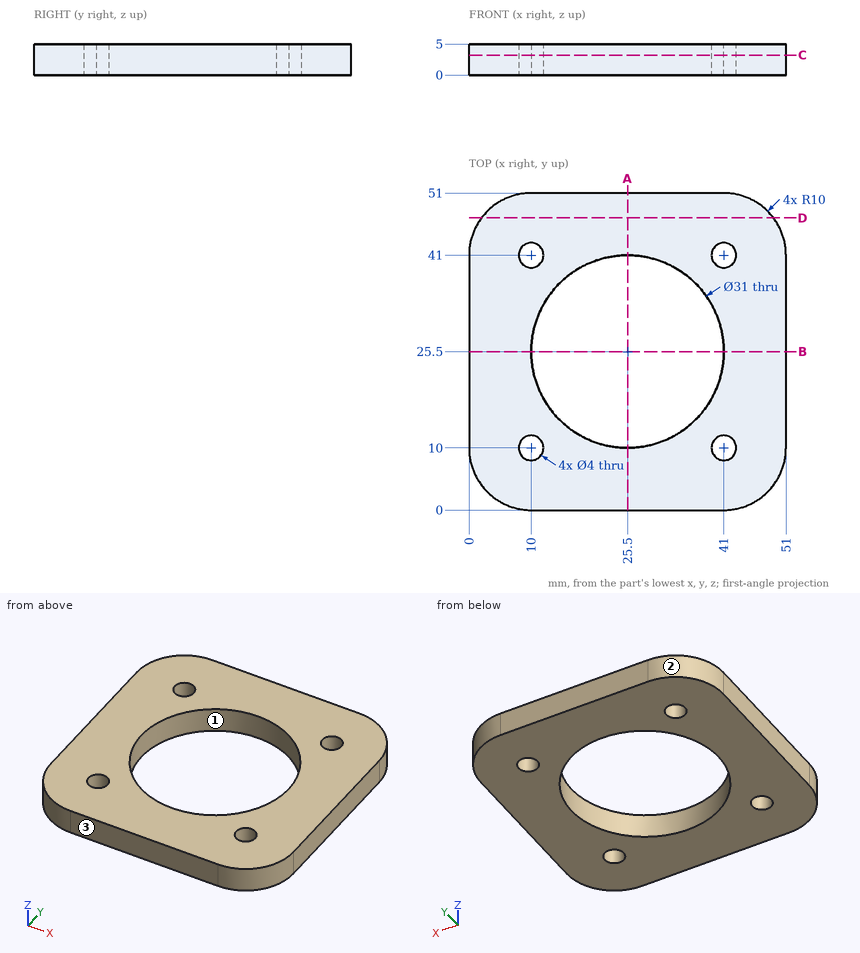
The drawing under review shows one solid part. Ordinate dimensions are in mm from its lowest x, y, z. Coordinates: 2 decimals unless noted, no trailing zeros. Write each loop counter-clockwise with the first axis right and the second up, starting at its lowest first coordinate (ties: lowest second). Pieces come first, ordered by that corner, then holes.
1) Add section C-C (z = 3.2). Write out the cut boundary in (x, y), plus the area to 3 significant figures.
2) Mouldability with a two-part tool opening along X and no side actions: class the marked faces 1, 2 and 3 as +X half, -X half, draft (parallel to the pull), parting line (faces both ways), or undercut.
3) To check wall thickness, follow L1, parallel to Y at x = 8.5, z = 1.35; L2, parallel to Y at x = 25.5, z = 3.3; L3, parallel to Y at x = 9.5, z = 4.5. State the ranges of each line that lie inside material, in increasing order.
4) Add section A-A (x = 25.5). Write out the cut boundary in (y, z), plus the area to 3 significant figures.
5) Add section D-D (y = 47). Write out the cut boundary in (x, z), plus the area to 3 significant figures.
Check result:
1. outline: (0, 10) arc R10 ccw to (10, 0) - (41, 0) arc R10 ccw to (51, 10) - (51, 41) arc R10 ccw to (41, 51) - (10, 51) arc R10 ccw to (0, 41) - close; hole circle Ø4 at (10, 10); hole circle Ø4 at (10, 41); hole circle Ø31 at (25.5, 25.5); hole circle Ø4 at (41, 10); hole circle Ø4 at (41, 41)
1. area: 1,710 mm2
2. face 1: undercut
2. face 2: -X half
2. face 3: draft
3. L1: y = 0.11 to 8.68, 11.32 to 39.68, 42.32 to 50.89
3. L2: y = 0 to 10, 41 to 51
3. L3: y = 0.01 to 8.06, 11.94 to 39.06, 42.94 to 50.99
4. outline: (0, 0) - (10, 0) - (10, 5) - (0, 5) - close; (41, 0) - (51, 0) - (51, 5) - (41, 5) - close
4. area: 100 mm2
5. outline: (2, 0) - (49, 0) - (49, 5) - (2, 5) - close
5. area: 235 mm2
